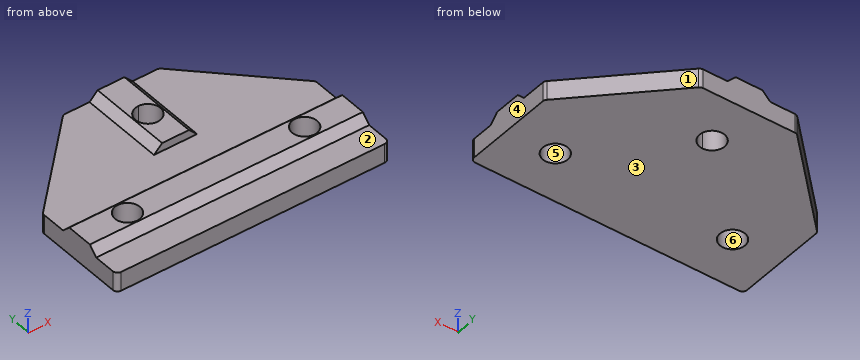
```python
from build123d import *

# Parameters (mm, degrees)
F0_R     = 2.6
F1_DEPTH = 4
F2_W     = 28.5
F2_H     = 9
F2_R     = 2.6
F3_DEPTH = 1.7
F4_SIZE  = 1.69999
F5_R     = 1


# Not quite as in the source:
# - a fillet or chamfer is up to 0.001 mm smaller than in the source, because OpenCascade refuses the exact size


with BuildPart() as f1:
    # F0 (on Top) → F1 (new body)
    with BuildSketch(Plane.XY):
        with BuildLine():
            Line((-28.5, 0), (0, 0))
            Line((0, 0), (0, 25.9))
            ThreePointArc((0, 25.9), (-2.6, 28.5), (0, 31.1))
            Line((0, 31.1), (0, 38.5))
            Line((0, 38.5), (-10, 38.5))
            Line((-10, 38.5), (-28.5, 20))
            Line((-28.5, 20), (-28.5, 0))
        make_face()
        with Locations((-18.5, 10)):
            Circle(F0_R, mode=Mode.SUBTRACT)
    extrude(amount=F1_DEPTH)

    # F2 (on face) → F3 (join)
    with BuildSketch(Plane.XY.offset(4)):
        with Locations((-14.25, 10)):
            Rectangle(F2_W, F2_H)
        with Locations((-18.5, 10)):
            Circle(F2_R, mode=Mode.SUBTRACT)
        with BuildLine():
            ThreePointArc((0, 25.9), (-2.6, 28.5), (0, 31.1))
            Line((0, 31.1), (0, 38.5))
            Line((0, 38.5), (-4.5, 38.5))
            Line((-4.5, 38.5), (-4.5, 21))
            Line((-4.5, 21), (0, 21))
            Line((0, 21), (0, 25.9))
        make_face()
    extrude(amount=F3_DEPTH)

    # F4 (size 1.7 in the source; OpenCascade refuses exactly that, so slightly less here)
    f4_edges = [f1.edges().sort_by_distance(p)[0] for p in [
        (-14.25, 14.5, 5.7),
        (-14.25, 5.5, 5.7),
        (-4.5, 29.75, 5.7),
    ]]
    chamfer(f4_edges, length=F4_SIZE)

    # F5
    f5_edges = [f1.edges().sort_by_distance(p)[0] for p in [
        (-10, 38.5, 2),
        (-28.5, 20, 2),
        (-28.5, 0, 2),
    ]]
    fillet(f5_edges, radius=F5_R)

    # F6: F1 across face


with BuildPart() as f1_1:
    add(f1.part)
    add(f1.part.mirror(Plane(origin=(0, 34.8, 2.85), x_dir=(0, 1, 0), z_dir=(1, 0, 0))))


solid = f1_1.part
```
Work out the finished part from the listing and answer in its coordinate system (mm). Face numbers are marked on the shaded views. A direction names the side the tool comes from. Give positions to 0.01 mm unless a question says otherwise; leave off trailing zeros. Loops run counter-clockwise (first coordinate to the right, second up) from the corner with the lowest first, then second, coordinate; pieces in that order, holes last. Notation, with made-up numbers: (0.25, 37.25) -> (49.25, 37.25) arc R16 cw to (49.25, 51.25) -> close; hole circle Ø3 at (-11.5, 2.5). An arc over 180 degrees is marked (long way). One line per question, with ' | ' between items. Start each with the question number.
1) Straight lines are drawn through the part: L1, parallel to X at y = 12, z = 2.1; L2, parallel to X at y = 11, z = 1.3; L3, parallel to Y at x = 18.5, z = 2.45. For each, find the intervals that lie inside material, in ascending order.
2) Determine the mould class of the marked faces 3, 4, 5 and 6 for opening direction X: +X half, -X half, draft (parallel to the pull), parting line (faces both ways), or undercut.
3) Section B-B, the plane y = 10 is taken. Determine the outline of the cut face in (x, z), then the cut area to 3 significant figures.
4) Section C-C, the plane z = 4.85 is taken. Determine the outline of the cut face in (x, y), then the cut area to 3 significant figures.
5) Each of these flat-tipped pins is pushed along its axis until it touches: pin 1 (4 mm diameter, centred on x = 21.5, y = 26.5, fed in from +Z); pin 2 (3 mm diameter, centred on y = 26, z = 0.5, fed in from -X); pin 3 (2 mm diameter, centred on y = 23, z = 1, fed in from -X). Where does it stop, or does it pass through?
6) For the marked faces 1 and 2, determine the directions among +Z, -Z, +X, -X, +Y, -Y from which every point of the face is accessible in a straight line to the end or side of a thin tool.
Resolved:
1) L1: -28.5 to -20.16, -16.84 to 16.84, 20.16 to 28.5 | L2: -28.5 to -20.9, -16.1 to 16.1, 20.9 to 28.5 | L3: 0 to 7.4, 12.6 to 30
2) face 3: draft | face 4: +X half | face 5: undercut | face 6: undercut
3) outline: (-28.5, 0) -> (-21.1, 0) -> (-21.1, 5.7) -> (-28.5, 5.7) -> close; (-15.9, 0) -> (15.9, 0) -> (15.9, 5.7) -> (-15.9, 5.7) -> close; (21.1, 0) -> (28.5, 0) -> (28.5, 5.7) -> (21.1, 5.7) -> close | area: 266 mm2
4) outline: (-28.5, 6.35) -> (28.5, 6.35) -> (28.5, 13.65) -> (-28.5, 13.65) -> close; (-3.65, 21) -> (3.65, 21) -> (3.65, 38.5) -> (-3.65, 38.5) -> close; hole circle Ø5.2 at (-18.5, 10); hole circle Ø5.2 at (0, 28.5); hole circle Ø5.2 at (18.5, 10) | area: 480 mm2
5) pin 1: z = 4 | pin 2: x = -24 | pin 3: x = -26.5
6) face 1: +Z, -Z, +X, +Y | face 2: +Z, +X, -X, -Y
